Autodesk Inventor part; units mm, degrees
ref_plane "YZ Plane" through (0, 0, 0) normal (1, 0, 0) x (0, 1, 0)
ref_plane "XZ Plane" through (0, 0, 0) normal (0, 1, 0) x (-1, 0, 0)
ref_plane "XY Plane" through (0, 0, 0) normal (0, 0, 1) x (1, 0, 0)
sketch "Sketch1" plane through (0, 0, 0) normal (0, 0, 1) x (1, 0, 0)
  line L0 (0, 0) -> (55, 0)
  line L1 (0, 0) -> (-76, 0)
  line L2 (-116, 0) -> (-138, 0)
  line L3 (-138, 0) -> (-138, 70)
  line L4 (-138, 70) -> (-138, 85)
  line L5 (-138, 85) -> (-116, 85)
  line L6 (-116, 0) -> (-116, 70)
  line L7 (-116, 70) -> (-76, 70)
  line L8 (-76, 70) -> (-76, 0)
  line L9 (90, 70) -> (90, 85)
  line L10 (90, 85) -> (-116, 85)
  line L11 (55, 0) -> (55, 70)
  line L12 (55, 70) -> (90, 70)
  line L13 (55, 0) -> (-76, 0)
  line L14 (-116, 0) -> (-117.6, 0)
  line L15 (-117.6, 0) -> (-117.6, 71.4164)
  line L16 (-117.6, 71.4164) -> (-74.4045, 71.4164)
  line L17 (-74.4045, 71.4164) -> (-74.4045, 0)
  line L18 (-138, 0) -> (-152.8138, 0)
  line L19 (-152.8138, 0) -> (-152.8138, 85)
  line L20 (-152.8138, 85) -> (-138, 85)
  dimension "d20" = 1.6
extrude "Extrusion1" add sketch "Sketch1" along normal blind 50 contours L1 L17 L16 L15 L2 L3 L4 L5 L10 L9 L12 L11 L0 | L1 L8 L7 L6 L2 L15 L16 L17
sketch "Sketch2" plane through (0, 0, 0) normal (1, 0, 0) x (0, 1, 0)
  point P0 (0, 0)
sketch "Sketch3" plane through (-76, 0, 0) normal (0, -1, 0) x (1, 0, 0)
  line L0 (131, 0) -> (131, 50)
  line L1 (131, 25) -> (76, 25)
  circle A0 centre (76, 25) radius 2.5
  point P0 (76, 0)
  dimension "d9" = 5
extrude "Extrusion2" cut sketch "Sketch3" against normal blind 50
sketch "Sketch4" plane through (55, 0, 0) normal (1, 0, 0) x (0, 0, -1)
  line L0 (0, 0) -> (-50, 0)
  circle A0 centre (-25, 0) radius 4.4
  dimension "d12" = 8.8
extrude "Extrusion3" cut sketch "Sketch4" against normal blind 238.5
sketch "Sketch5" plane through (55, 0, 0) normal (1, 0, 0) x (0, 0, -1)
  arc A0 (-20.6, 0) -> (-29.4, 0) centre (-25, 0) ccw
  circle A1 centre (-25, 0) radius 8
  circle A2 centre (-25, 0) radius 4.4
  point P0 (0, 0)
  dimension "d15" = 16
extrude "Extrusion4" add sketch "Sketch5" against normal up to surface (193 mm away)
sketch "Sketch6" plane through (0, 0, 50) normal (0, 0, 1) x (1, 0, 0)
  line L0 (-116, 0) -> (-116, 70)
  line L1 (-116, 13.3517) -> (-76, 13.3517)
  line L2 (-76, 13.3517) -> (-76, -16.9742)
  line L3 (-76, -16.9742) -> (-116, -16.9742)
  line L4 (-116, -16.9742) -> (-116, 13.3517)
  point P0 (0, 0)
extrude "Extrusion5" cut sketch "Sketch6" against normal blind 238.5
properties part number "Arm_Base"
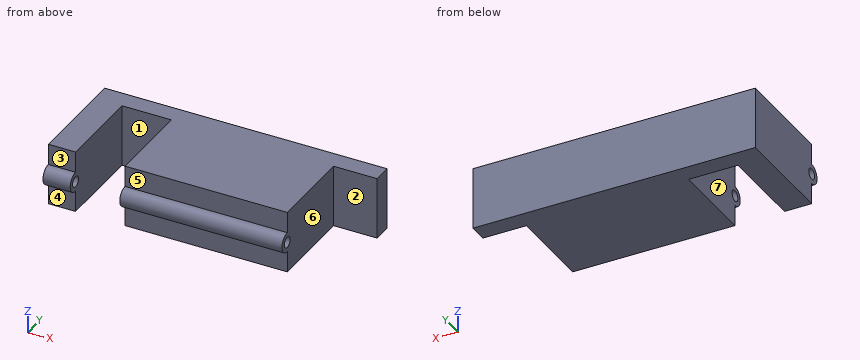
CAD build for the part. Positions are in the model's coordinates, mm. Face numbers are marked on the shaded views. A direction names the side the tool comes from. Coordinates: 2 decimals unless noted, no trailing zeros. Write each loop counter-clockwise with the first axis right and the second up, starting at its lowest first coordinate (ties: lowest second). Pieces come first, ordered by that corner, then holes. Notation, with made-up numbers: (4.5, 75) -> (30.5, 75) arc R29 ccw to (30.5, 102) -> close; hole circle Ø2 at (18.5, 11). An arc over 180 degrees is marked (long way). Return JSON: item names as keys, results as strings. Group by question number.
Q1. Which spindle directions (+Z, -Z, +X, -X, +Y, -Y) get a long thin tool onto all of the face, cutting with end or side? Do the marked faces 1, 2, 3 and 4. Say none if no direction does.
Q2. Drill centre lines: line 1 (X direction, y = 25, z = 25); line 2 (X direction, y = 34.5, z = 14); line 3 (Y direction, x = 1, z = 25). Where is each one in solid material? Low to high.
Q3. Cut at C-C, the plane x = 0. Give the cut face in (y, z).
Q4. Flat gauge pins, fed straight in: pin 1 (6 mm diameter, centred on x = 55.5, z = 38, fed in from -Y); pin 2 (6 mm diameter, centred on y = 34, z = 11.5, fed in from +X); pin 3 (8 mm diameter, centred on y = 0, z = 25, fed in from +X); pin 4 (10.5 mm diameter, centred on x = 81, z = 18.5, fed in from -Y). Where does each tip first touch, or does it go through?
Q5. Pull direction X, two halves, no side cores. Call the marked faces 5, 6 and 7: released by +X, released by -X, zero draft, split by the parting line, or undercut.
Q6. Cut at D-D, the plane y = 62. Give the cut face in (x, z), then the cut area to 3 significant figures.
Q7. Cut at A-A, the plane y = 36.5. Give the cut face in (x, z), then the cut area to 3 significant figures.
Q8. Cut at B-B, the plane z = 25. Give the cut face in (x, y), then the cut area to 3 significant figures.
Returned:
{
 "1": {"face 1": "+Z, -Z, -Y", "face 2": "+Z, -Z, +X, -Y", "face 3": "+Z, +X, -X, -Y", "face 4": "-Z, +X, -X, -Y"},
 "2": {"line 1": "x = -138 to -116, -76 to -2.5, 2.5 to 55", "line 2": "x = -138 to -116, -76 to 55", "line 3": "y = -8 to -4.4, 4.4 to 8, 50 to 85"},
 "3": {"outline": "(0, 0) -> (85, 0) -> (85, 50) -> (0, 50) -> (0, 33) arc R8 ccw to (0, 17) -> close; hole circle Ø8.8 at (0, 25); hole (7.6, 22.5) -> (50, 22.5) -> (50, 27.5) -> (7.6, 27.5) arc R8 cw to start"},
 "4": {"pin 1": "stops at y = 0", "pin 2": "stops at x = 55", "pin 3": "passes through", "pin 4": "stops at y = 70"},
 "5": {"face 5": "zero draft", "face 6": "released by +X", "face 7": "undercut"},
 "6": {"outline": "(-138, 0) -> (-116, 0) -> (-116, 50) -> (-138, 50) -> close; (-76, 0) -> (55, 0) -> (55, 50) -> (-76, 50) -> close", "area": "7,650 mm2"},
 "7": {"outline": "(-138, 0) -> (-116, 0) -> (-116, 50) -> (-138, 50) -> close; (-76, 0) -> (55, 0) -> (55, 50) -> (-76, 50) -> close; hole circle Ø5 at (0, 25)", "area": "7,630 mm2"},
 "8": {"outline": "(-138, -8) -> (-116, -8) -> (-116, -4.4) -> (-138, -4.4) -> close; (-138, 4.4) -> (-116, 4.4) -> (-116, 70) -> (-76, 70) -> (-76, 4.4) -> (55, 4.4) -> (55, 70) -> (90, 70) -> (90, 85) -> (-138, 85) -> close; (-76, -8) -> (55, -8) -> (55, -4.4) -> (-76, -4.4) -> close; hole (-2.5, 8) -> (2.5, 8) -> (2.5, 50) -> (-2.5, 50) -> close", "area": "13,800 mm2"}
}
